Here's how the part is built. I have some questions about the finished solid (model axes, mm). A direction names the side the tool comes from. Round coordinates to 2 decimals unless told otherwise and drop trailing zeros. Order: outer loops, then holes, each group sorted by start corner. A loop starts at its lowest first (then second) coordinate and runs counter-clockwise, first axis right, second up. Notation, with made-up numbers: M -33.5,10.25 L 5.5,10.25 A30 cw 5.5,46.25 Z; hole C 78,50.5 d7. An arc over 180 degrees is marked long. Write item = value, one per line. Start each with the question number.
Item 1: Please list where these lines run through material, in increasing order: L1, parallel to Y at x = 33, z = -22.25; L2, parallel to X at y = 12.5, z = -20.25; L3, parallel to X at y = 21.75, z = -18.5.
Item 2: I want a section at D-D, the plane z = -18. State how many separate pieces and enclosed holes the cut face has, plus the area to 3 significant figures.
Item 3: I want a section at B-B, the plane x = 12.5. List the corners of the cut face in (y, z) for me, plus the area to 3 significant figures.
Item 4: I want a section at A-A, the plane y = 7. List the corners of the cut face in (x, z) for me.
Item 5: I want a section at C-C, the plane y = 3. List the corners of the cut face in (x, z) for me.
Item 6: I'm going to push flat-ended pins straight in: P1, Ø2.5, axis at x = 13.5, z = -14, coming from the -Y side; P2, Ø8, axis at x = 31.5, z = -16, coming from the +Y side; P3, Ø0.6, axis at x = 16, z = 1.5, coming from the +Y side. Where does each tip first touch, or does it pass through?
Item 7: For faces 1 (the face through (-5, 2, -11)), 2 (the face through (0, 6, -12)), 3 (the face through (6.5, 7, 1)), 4 (the face through (30.71, 0.99, -18.99)), 5 (the face through (29, 7, -11)), which set-ups out of +Z, -Z, +X, -X, +Y, -Y let a thin tool reach every point of the face, with its end or its side?
Item 8: We'd pull the mould along X, two halves only. Please class faces 6 (the face through (24.8, 21, -11.3)), 7 (the face through (13, 4.5, 1)), 8 (the face through (13, 25, -11)): pulls with the +X half, pulls with the -X half, needs draft (parallel to the pull), parting line crosses it, or undercut.
```python
from build123d import *

# Parameters (mm, degrees)
F0_W     = 14
F0_H     = 6
F1_DEPTH = 2
F3_DEPTH = 25
F4_R     = 1.625
F5_DEPTH = 2


with BuildPart() as f1:
    # F0 (on Top) → F1 (new body)
    with BuildSketch(Plane.XY):
        with BuildLine():
            ThreePointArc((0, 11), (3.5147186258, 19.4852813742), (12, 23))
            Line((12, 23), (15, 23))
            ThreePointArc((15, 23), (23.4852813742, 19.4852813742), (27, 11))
            Line((27, 11), (27, 5))
            Line((27, 5), (27, 0))
            Line((27, 0), (29, 0))
            Line((29, 0), (29, 5))
            Line((29, 5), (29, 11))
            ThreePointArc((29, 11), (24.8994949366, 20.8994949366), (15, 25))
            Line((15, 25), (12, 25))
            ThreePointArc((12, 25), (2.1005050634, 20.8994949366), (-2, 11))
            Line((-2, 11), (-2, 5))
            Line((-2, 5), (-2, 0))
            Line((-2, 0), (0, 0))
            Line((0, 0), (0, 5))
            Line((0, 5), (0, 11))
        make_face()
        with BuildLine():
            Line((15, 23), (12, 23))
            ThreePointArc((12, 23), (3.5147186258, 19.4852813742), (0, 11))
            Line((0, 11), (0, 5))
            Line((0, 5), (0, 0))
            Line((0, 0), (27, 0))
            Line((27, 0), (27, 5))
            Line((27, 5), (27, 11))
            ThreePointArc((27, 11), (23.4852813742, 19.4852813742), (15, 23))
        make_face()
        with Locations((13.5, 7.5)):
            Rectangle(F0_W, F0_H, mode=Mode.SUBTRACT)
    extrude(amount=F1_DEPTH)

    # F2 (on face) → F3 (join)
    with BuildSketch(Plane(origin=(0, 0, 0), x_dir=(1, 0, 0), z_dir=(0, 0, -1))):
        with BuildLine():
            Line((0, -11), (0, 0))
            Line((0, 0), (-2, 0))
            Line((-2, 0), (-2, -11))
            ThreePointArc((-2, -11), (2.1005050634, -20.8994949366), (12, -25))
            Line((12, -25), (15, -25))
            ThreePointArc((15, -25), (24.8994949366, -20.8994949366), (29, -11))
            Line((29, -11), (29, 0))
            Line((29, 0), (27, 0))
            Line((27, 0), (27, -11))
            ThreePointArc((27, -11), (23.4852813742, -19.4852813742), (15, -23))
            Line((15, -23), (12, -23))
            ThreePointArc((12, -23), (3.5147186258, -19.4852813742), (0, -11))
        make_face()
    extrude(amount=F3_DEPTH)

    # F4 (on face) → F5 (join)
    with BuildSketch(Plane.XZ):
        with BuildLine():
            add(Edge.make_bspline(
                [(29, 2), (33.0137730771, -5.6907851712), (39.7482218864, -18.594653438), (32.0927595214, -23.1568861551), (29, -25)],
                knots=[0, 0, 0, 0, 0.5960061752, 1, 1, 1, 1], degree=3))
            Line((29, 2), (29, -25))
        make_face()
        with Locations((32, -18)):
            Circle(F4_R, mode=Mode.SUBTRACT)
        with BuildLine():
            Line((-2, -25), (-2, 2))
            add(Edge.make_bspline(
                [(-2, 2), (-6.0137730771, -5.6907851712), (-12.7482218864, -18.594653438), (-5.0927595214, -23.1568861551), (-2, -25)],
                knots=[0, 0, 0, 0, 0.5960061752, 1, 1, 1, 1], degree=3))
        make_face()
        with Locations((-5, -18)):
            Circle(F4_R, mode=Mode.SUBTRACT)
    extrude(amount=-F5_DEPTH)


solid = f1.part
```
Filled in:
q1.L1 = 0 to 2
q1.L2 = -1.92 to 0.09, 26.91 to 28.92
q1.L3 = 3.03 to 6.67, 20.33 to 23.97
q2.separate_pieces = 3
q2.enclosed_holes = 0
q2.area = 146 mm^2
q3.outline = M 0,0 L 4.5,0 L 4.5,2 L 0,2 Z; M 10.5,0 L 23,0 L 23,-25 L 25,-25 L 25,2 L 10.5,2 Z
q3.area = 88.0 mm^2
q4.outline = M -2,-25 L 0,-25 L 0,0 L 6.5,0 L 6.5,2 L -2,2 Z; M 20.5,0 L 27,0 L 27,-25 L 29,-25 L 29,2 L 20.5,2 Z
q5.outline = M -2,-25 L 0,-25 L 0,0 L 27,0 L 27,-25 L 29,-25 L 29,2 L -2,2 Z
q6.P1 = 23
q6.P2 = 17.3
q6.P3 = 24.98
q7.face_1 = +Z, -Z, -X, +Y
q7.face_2 = -Z, -Y
q7.face_3 = +Z, -Z
q7.face_4 = +Y, -Y
q7.face_5 = +Z, -Z, +X, +Y
q8.face_6 = pulls with the +X half
q8.face_7 = undercut
q8.face_8 = needs draft
